Design review of the part shown in the three views and the two pictorial views. Dimensions are in mm from the part's minimum x, y and z. Round coordinates to 2 decimals unless told otherwise and drop trailing zeros. Order: outer loops, then holes, each group sorted by start corner. A loop starts at its lowest first (then second) coordinate and runs counter-clockwise, first axis right, second up. Notation, with made-up numbers: M -9.5,54 L 10.5,54 A33 ccw 10.5,84 Z; hole C 21,26.5 d2. An arc over 180 degrees is marked long. Write each question's results on one line, items separated by ' | '. Start each with the question number.
Item 1: Wall thickness on line 1 (Z direction, x = 69.85, y = 2) (1 decimal); line 2 (X direction, y = 5, z = 59) (1 decimal); line 3 (Y direction, x = 14.5, z = 44): over which ranges is each line inside the solid? List them lowest first. Write a range as [from, to].
Item 2: The part is to be moulded in two halves that separate along X. For the marked faces 1, 2 and 3, say which applies: +X half, -X half, draft (parallel to the pull), parting line (faces both ways), or undercut.
Item 3: Take a section at B-B, the plane y = 14.5. Write out the cut boundary in (x, z) (1 decimal).
Item 4: Take a section at C-C, the plane z = 69.85. Count the separate pieces of the cut face and the enclosed holes in it.
Item 5: Clearance check with flat-ended pins moving along their axes: pin 1 (2 mm diameter, centred on x = 15.494, z = 60.706, fed in from -Y); pin 2 (9 mm diameter, centred on x = 69.85, z = 69.85, fed in from +Y); pin 3 (1 mm diameter, centred on x = 67, z = 29, fed in from -Y); pin 4 (6.5 mm diameter, centred on x = 19.05, y = 11.11, fed in from -Z) (1 decimal). State where each tip first meets the part, or that it passes through.
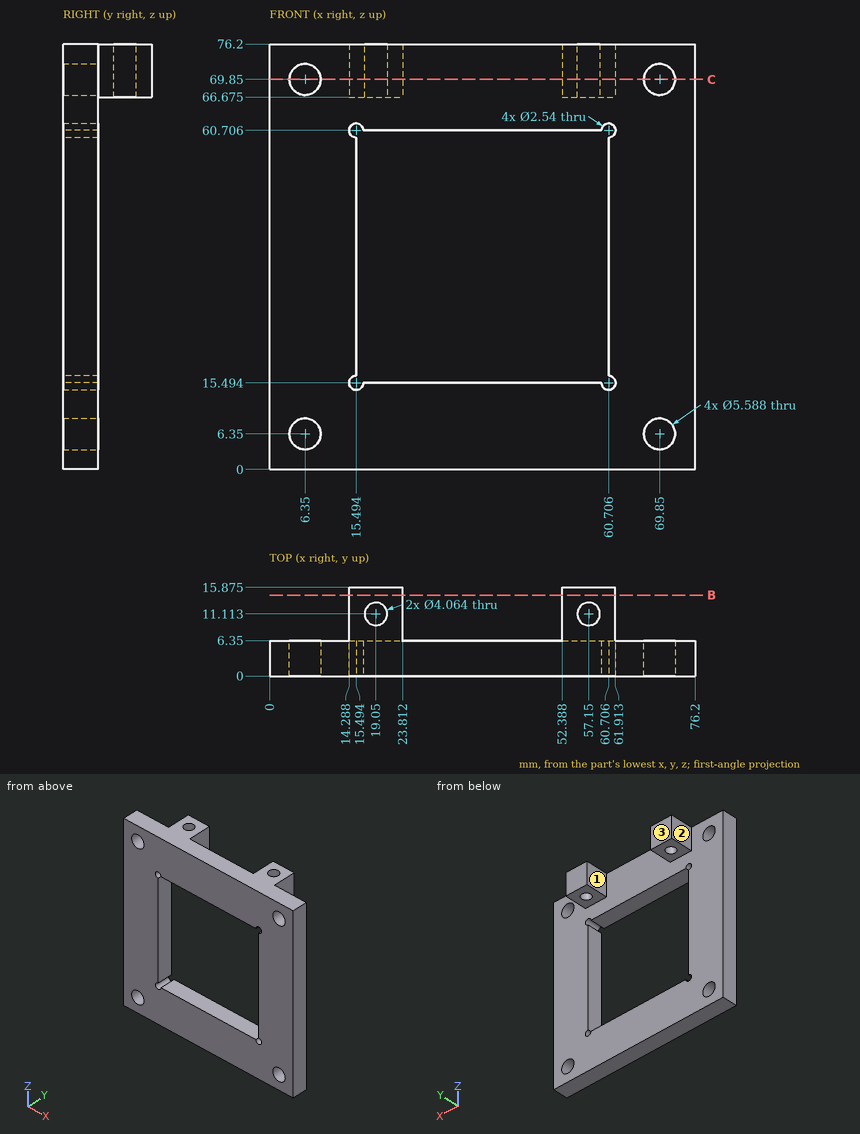
Results list:
1) line 1: [0, 3.6], [9.1, 67.1], [72.6, 76.2] | line 2: [0, 15.5], [60.7, 76.2] | line 3: [0, 6.35]
2) face 1: undercut | face 2: -X half | face 3: draft
3) outline: M 14.3,66.7 L 23.8,66.7 L 23.8,76.2 L 14.3,76.2 Z; M 52.4,66.7 L 61.9,66.7 L 61.9,76.2 L 52.4,76.2 Z
4) separate pieces: 3 | enclosed holes: 2
5) pin 1: through | pin 2: y = 6.35 | pin 3: y = 0 | pin 4: z = 66.7
